```python
from build123d import *

# Parameters (mm, degrees)
SKETCH1_W           = 20
SKETCH1_H           = 10
BOSS_EXTRUDE1_DEPTH = 4
SKETCH4_W           = 14.741858766
SKETCH4_H           = 10
BOSS_EXTRUDE3_DEPTH = 2
CUT_EXTRUDE2_DEPTH  = 10
SKETCH6_R           = 1.25
CUT_EXTRUDE3_DEPTH  = 10
FILLET1_R           = 2


with BuildPart() as part:
    # Sketch1 → Boss-Extrude1 (new body)
    with BuildSketch(Plane(origin=(0, 0, 0), x_dir=(1, 0, 0), z_dir=(0, 1, 0))):
        Rectangle(SKETCH1_W, SKETCH1_H)
    extrude(amount=BOSS_EXTRUDE1_DEPTH)

    # Sketch4 → Boss-Extrude3 (add)
    with BuildSketch(Plane(origin=(0, 4, 0), x_dir=(1, 0, 0), z_dir=(0, 1, 0))):
        Rectangle(SKETCH4_W, SKETCH4_H)
    extrude(amount=BOSS_EXTRUDE3_DEPTH)

    # Sketch5 → Cut-Extrude2 (cut)
    with BuildSketch(Plane.XY.offset(5)):
        Polygon((0, 3.998182385), (0, 6), (-1.5, 6), (-2, 6), align=None)
        Polygon((1.5, 6), (0, 6), (0, 3.998182385), (2, 6), align=None)
    extrude(amount=-CUT_EXTRUDE2_DEPTH, mode=Mode.SUBTRACT)

    # Sketch6 → Cut-Extrude3 (cut)
    with BuildSketch(Plane(origin=(0, 6, 0), x_dir=(1, 0, 0), z_dir=(0, 1, 0))):
        with Locations(Location((-4.685464692, 0, 0), (0, 0, 270))):
            Circle(SKETCH6_R)
        with Locations(Location((4.685464692, 0, 0), (0, 0, 270))):
            Circle(SKETCH6_R)
    extrude(amount=-CUT_EXTRUDE3_DEPTH, mode=Mode.SUBTRACT)

    # Fillet1
    fillet1_edges = [part.edges().sort_by_distance(p)[0] for p in [
        (-7.370929383, 4, 0),
        (7.370929383, 4, 0),
    ]]
    fillet(fillet1_edges, radius=FILLET1_R - 0.0001)  # a hair under: the kernel refuses the full size


solid = part.part
```
Verification items for the finished model (mm, model axes). A direction names the side the tool comes from. Round coordinates to 2 decimals unless told otherwise and drop trailing zeros. Loops run counter-clockwise (first coordinate to the right, second up) from the corner with the lowest first, then second, coordinate; pieces in that order, holes last. Notation, with made-up numbers: (70, 68.25) -> (89, 68.25) arc R23 ccw to (89, 90.25) -> close; hole circle Ø1 at (4, -33.5). An arc over 180 degrees is marked (long way). Answer as a JSON object with one key per item and string values.
Q1. Section check A-A (z = 0). State how many separate pieces and enclosed holes the cut face has, then the cut area to 3 significant figures.
Data:
{"separate pieces": "3", "enclosed holes": "0", "area": "77.2 mm2"}
Q2. Go/stop test with a flat-tipped pin: P1, Ø2, axis at x = 4.69, z = 0, coming from the -Y side. Record where the tip stops, or that it passes through.
Data:
{"P1": "passes through"}
Q3. Scan lines: line 1 (X direction, y = 3.6, z = 0); line 2 (Z direction, x = 4.75, y = 5.7); line 3 (X direction, y = 5.1, z = -0.5). Record each from-to range of solid material in increasing order. Write a range as from..to.
Data:
{"line 1": "x = -10..-5.94, -3.44..3.44, 5.94..10", "line 2": "z = -5..-1.25, 1.25..5", "line 3": "x = -7.58..-5.83, -3.54..-1.1, 1.1..3.54, 5.83..7.58"}
Q4. Section check B-B (y = 5.35). Record the boundary of the cut face in (x, z).
Data:
{"outline": "(-7.48, -5) -> (-1.35, -5) -> (-1.35, 5) -> (-7.48, 5) -> close; (1.35, -5) -> (7.48, -5) -> (7.48, 5) -> (1.35, 5) -> close; hole circle Ø2.5 at (-4.69, 0); hole circle Ø2.5 at (4.69, 0)"}
Q5. Draft check along Z on faces 3 (the cylindrical face through (5.925, 3.042, -0.163)), 4 (the cylindrical face through (-5.9, 3, -0.3)), 5 (the flat face through (0, 3, 5)), 6 (the flat face through (1, 5, 0)). Enter one of: pulls with the +Z half, pulls with the -Z half, needs draft (parallel to the pull), parting line crosses it, or undercut.
Data:
{"face 3": "undercut", "face 4": "undercut", "face 5": "pulls with the +Z half", "face 6": "needs draft"}
Q6. Access from +Z, -Z, +X, -X, +Y, -Y to the whole of each face (thin tool, end or side, straight path). Record for faces 1 (the flat face through (-1, 5, 0)), 2 (the cylindrical face through (-7.97, 4.57, -0.07)).
Data:
{"face 1": "+Z, -Z, +Y", "face 2": "+Z, -Z, -X, +Y"}
Q7. Section check C-C (x = 4.5). Record the boundary of the cut face in (y, z).
Data:
{"outline": "(0, -5) -> (6, -5) -> (6, -1.24) -> (0, -1.24) -> close; (0, 1.24) -> (6, 1.24) -> (6, 5) -> (0, 5) -> close"}
